```python
from build123d import *

# Parameters (mm, degrees)
SKETCH_1_R          = 24
SKETCH_1_R_2        = 2
SKETCH_1_R_3        = 2.5
SKETCH_1_R_4        = 1.1
SKETCH_1_R_5        = 6
EXTRUDE_1_DEPTH     = 4
SKETCH_2_R          = 1
CUT_EXTRUDE_1_DEPTH = 84.312664103
CUT_EXTRUDE_2_DEPTH = 10
FILLET_2_R          = 2
FILLET_3_R          = 2


with BuildPart() as part:
    # 草图1 → 凸台-拉伸1 (new body)
    with BuildSketch(Plane.XY):
        with BuildLine():
            Line((-31, 0), (-31, 44.038518603))
            ThreePointArc((-31, 44.038518603), (-32.603168898, 47.707515532), (-36.384615385, 49.023703756))
            ThreePointArc((-36.384615385, 49.023703756), (-44.994071865, 56.692079518), (-37, 65))
            Line((-37, 65), (-12.5, 65))
            Line((-12.5, 65), (-12.5, 70))
            Line((-12.5, 70), (12.5, 70))
            Line((12.5, 70), (12.5, 65))
            Line((12.5, 65), (31, 65))
            Line((31, 65), (31, 0))
            ThreePointArc((31, 0), (24.191352338, -19.385006373), (6.756227609, -30.254807692))
            ThreePointArc((6.756227609, -30.254807692), (5.147421514, -30.170867126), (3.813999457, -29.266826923))
            ThreePointArc((3.813999457, -29.266826923), (0, -27.5), (-3.813999457, -29.266826923))
            ThreePointArc((-3.813999457, -29.266826923), (-5.147421514, -30.170867126), (-6.756227609, -30.254807692))
            ThreePointArc((-6.756227609, -30.254807692), (-24.191352338, -19.385006373), (-31, 0))
        make_face()
        Circle(SKETCH_1_R, mode=Mode.SUBTRACT)
        with Locations((-19.445436483, 19.445436483)):
            Circle(SKETCH_1_R_2, mode=Mode.SUBTRACT)
        with Locations((0, 27.5)):
            Circle(SKETCH_1_R_2, mode=Mode.SUBTRACT)
        with Locations((19.445436483, 19.445436483)):
            Circle(SKETCH_1_R_2, mode=Mode.SUBTRACT)
        with Locations((27.5, 0)):
            Circle(SKETCH_1_R_2, mode=Mode.SUBTRACT)
        with Locations((19.445436483, -19.445436483)):
            Circle(SKETCH_1_R_2, mode=Mode.SUBTRACT)
        with Locations((-19.445436483, -19.445436483)):
            Circle(SKETCH_1_R_2, mode=Mode.SUBTRACT)
        with Locations((-27.5, 0)):
            Circle(SKETCH_1_R_2, mode=Mode.SUBTRACT)
        with Locations((-26, 60)):
            Circle(SKETCH_1_R_3, mode=Mode.SUBTRACT)
        with Locations((0, 60)):
            Circle(SKETCH_1_R_3, mode=Mode.SUBTRACT)
        with Locations((26, 60)):
            Circle(SKETCH_1_R_3, mode=Mode.SUBTRACT)
        with Locations((-22.6, 50)):
            Circle(SKETCH_1_R_4, mode=Mode.SUBTRACT)
        with Locations((-22.6, 32)):
            Circle(SKETCH_1_R_4, mode=Mode.SUBTRACT)
        with Locations((22.6, 32)):
            Circle(SKETCH_1_R_4, mode=Mode.SUBTRACT)
        with Locations((22.6, 50)):
            Circle(SKETCH_1_R_4, mode=Mode.SUBTRACT)
        with Locations((-37, 57)):
            Circle(SKETCH_1_R_5, mode=Mode.SUBTRACT)
    extrude(amount=EXTRUDE_1_DEPTH)

    # 草图2 → 切除-拉伸1 (cut, through all)
    with BuildSketch(Plane.XY.offset(4)):
        with Locations((-13.5, 65)):
            Circle(SKETCH_2_R)
        with Locations((13.5, 65)):
            Circle(SKETCH_2_R)
    extrude(amount=-CUT_EXTRUDE_1_DEPTH, mode=Mode.SUBTRACT)

    # 草图3 → 切除-拉伸2 (cut)
    with BuildSketch(Plane.XY.offset(4)):
        with BuildLine():
            Line((-3, 54), (-17.6, 54))
            Line((-17.6, 54), (-17.6, 26.124509565))
            ThreePointArc((-17.6, 26.124509565), (-10.627053281, 29.653258482), (-3, 31.356817441))
            Line((-3, 31.356817441), (-3, 54))
        make_face()
        with BuildLine():
            Line((17.6, 54), (3, 54))
            Line((3, 54), (3, 31.356817441))
            ThreePointArc((3, 31.356817441), (10.627053281, 29.653258482), (17.6, 26.124509565))
            Line((17.6, 26.124509565), (17.6, 54))
        make_face()
    extrude(amount=-CUT_EXTRUDE_2_DEPTH, mode=Mode.SUBTRACT)

    # 圆角2
    fillet_2_edges = [part.edges().sort_by_distance(p)[0] for p in [
        (-3, 31.356817441, 2),
        (-17.6, 26.124509565, 2),
        (-17.6, 54, 2),
        (-3, 54, 2),
        (17.6, 26.124509565, 2),
        (3, 31.356817441, 2),
        (3, 54, 2),
        (17.6, 54, 2),
    ]]
    fillet(fillet_2_edges, radius=FILLET_2_R)

    # 圆角3
    fillet_3_edges = [part.edges().sort_by_distance(p)[0] for p in [
        (31, 65, 2),
    ]]
    fillet(fillet_3_edges, radius=FILLET_3_R)


solid = part.part
```
Model file for the job. Use its own axes, mm. A direction names the side the tool comes from. Coordinates: 2 decimals unless noted, no trailing zeros. Loops run counter-clockwise (first coordinate to the right, second up) from the corner with the lowest first, then second, coordinate; pieces in that order, holes last. Notation, with made-up numbers: M -8.75,30.25 L -1.75,30.25 A22 ccw -1.75,55.25 Z; hole C -6,-3.75 d6. An arc over 180 degrees is marked long. Use CSV: the item, a comma, the result in double quotes. Start each with the question number.
1. Two-plate mould, pull along X, no slides. Class faces 3 (the cylindrical face through (3.6, 53.43, 1.97)), 4 (the cylindrical face through (30.43, 64.4, 2.03)), 5 (the cylindrical face through (-24.01, -19.61, 1.97)): pulls with the +X half, pulls with the -X half, needs draft (parallel to the pull), parting line crosses it, or undercut.
2. Band-saw the part on A-A, the plane x = 0. List the corners of the cut face in (y, z), then the cut area to 3 significant figures.
3. Band-saw the part on B-B, the plane y = 41. List the corners of the cut face in (x, z), then the cut area to 3 significant figures.
4. Probe probe 1 along Y at (x, z) = (0, 2.8); probe 2 along Y at (x, z) = (21, 1.6); probe 3 along Y at (x, z) = (27.5, 2.4). List the from-to ranges inside material, lowest first. Write a range as [from, to].
5. Tool access for faces 1 (the cylindrical face through (-3.5, 31.8, 2)), 2 (the cylindrical face through (13.5, 64, 2)): list every direction of +Z, -Z, +X, -X, +Y, -Y with a clear straight run to the whole face (end or side of a thin tool).
6. Band-saw the part on C-C, the plane y = 8.5. List the corners of the cut face in (x, z).
7. Flat gauge pins, fed straight in: pin 1 (2 mm diameter, centred on y = 21, z = 2.5, fed in from -X); pin 2 (2 mm diameter, centred on y = 46, z = 1, fed in from -X); pin 3 (1.5 mm diameter, centred on x = 17, z = 0.5, fed in from +Y). Where does each tip first touch, or does it go through?
8. Band-saw the part on D-D, the plane x = -38.5. List the corners of the cut face in (y, z).
Entries:
1,face 3,"undercut"
1,face 4,"pulls with the +X half"
1,face 5,"pulls with the -X half"
2,outline,"M -27.5,0 L -24,0 L -24,4 L -27.5,4 Z; M 24,0 L 25.5,0 L 25.5,4 L 24,4 Z; M 29.5,0 L 57.5,0 L 57.5,4 L 29.5,4 Z; M 62.5,0 L 70,0 L 70,4 L 62.5,4 Z"
2,area,"162 mm2"
3,outline,"M -31,0 L -17.6,0 L -17.6,4 L -31,4 Z; M -3,0 L 3,0 L 3,4 L -3,4 Z; M 17.6,0 L 31,0 L 31,4 L 17.6,4 Z"
3,area,"131 mm2"
4,probe 1,"y = [-27.5, -24], [24, 25.5], [29.5, 57.5], [62.5, 70]"
4,probe 2,"y = [-22.8, -20.7], [-18.19, -11.62], [11.62, 18.19], [20.7, 65]"
4,probe 3,"y = [-14.31, -2], [2, 58], [62, 65]"
5,face 1,"+Z, -Z"
5,face 2,"+Z, -Z, +Y"
6,outline,"M -31,0 L -22.44,0 L -22.44,4 L -31,4 Z; M 22.44,0 L 31,0 L 31,4 L 22.44,4 Z"
7,pin 1,"stops at x = -31"
7,pin 2,"stops at x = -31.97"
7,pin 3,"stops at y = 65"
8,outline,"M 49.14,0 L 51.19,0 L 51.19,4 L 49.14,4 Z; M 62.81,0 L 64.86,0 L 64.86,4 L 62.81,4 Z"
